Check sheet for the drawn part. Datum: minimum x, y, z corner. Units: mm. Coordinates: 2 decimals unless noted, no trailing zeros. Order: outer loops, then holes, each group sorted by start corner. A loop starts at its lowest first (then second) coordinate and runs counter-clockwise, first axis right, second up. Notation, with made-up numbers: (-27, 77) -> (18, 77) arc R12 cw to (18, 89) -> close; hole circle Ø11 at (-32.5, 67). An arc over 180 degrees is marked (long way). Answer as CSV lines item,"result".
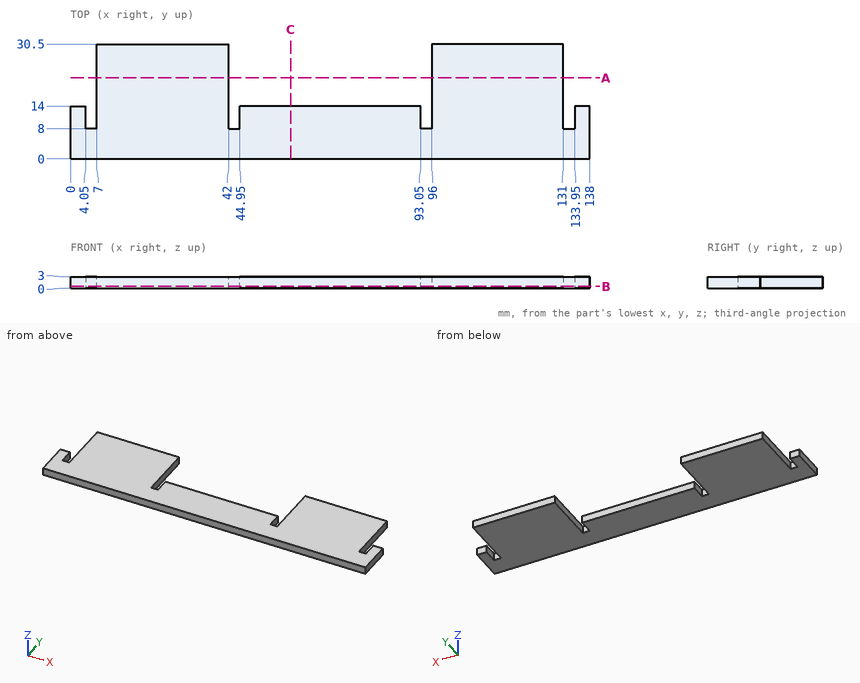
Item 1: Section check A-A, the plane y = 21.5. Record the boundary of the cut face in (x, z).
Answer list:
outline,"(7, 0) -> (42, 0) -> (42, 3) -> (7, 3) -> close; (96, 0) -> (131, 0) -> (131, 3) -> (96, 3) -> close"
Item 2: Thickness scan on line 1 (X direction, y = 12.5, z = 2.6); line 2 (X direction, y = 28.5, z = 0.8); line 3 (Y direction, x = 50.5, z = 1.7). Record the ranges inside material, lowest first.
Answer list:
line 1,"0 to 4.05, 7 to 42, 44.95 to 93.05, 96 to 131, 133.95 to 138"
line 2,"7 to 42, 96 to 131"
line 3,"0 to 14"
Item 3: Depth check by flat-ended pin: pin 1 Ø8 at (x, y) = (107.5, 3) entering from -Z; pin 2 Ø0.9 at (x, z) = (136, 1.5) entering from +Y; pin 3 Ø0.9 at (x, z) = (132, 1.5) entering from +Y; pin 4 Ø1.5 at (y, z) = (19.5, 1) entering from -X. Enter the tip coordinate at first touch or a pass-through.
Answer list:
pin 1,"z = 0"
pin 2,"y = 14"
pin 3,"y = 8"
pin 4,"x = 7"
Item 4: Section check B-B, the plane z = 0.45. Record the boundary of the cut face in (x, y), plus the area to 3 significant figures.
Answer list:
outline,"(0, 0) -> (138, 0) -> (138, 14) -> (133.95, 14) -> (133.95, 8) -> (131, 8) -> (131, 30.5) -> (96, 30.5) -> (96, 8) -> (93.05, 8) -> (93.05, 14) -> (44.95, 14) -> (44.95, 8) -> (42, 8) -> (42, 30.5) -> (7, 30.5) -> (7, 8) -> (4.05, 8) -> (4.05, 14) -> (0, 14) -> close"
area,"3,020 mm2"
Item 5: Section check C-C, the plane x = 58.5. Record the boundary of the cut face in (y, z), plus the area to 3 significant figures.
Answer list:
outline,"(0, 0) -> (14, 0) -> (14, 3) -> (0, 3) -> close"
area,"42.0 mm2"
